The drawing under review shows one solid part. Ordinate dimensions are in mm from its lowest x, y, z. Give positions to 0.01 mm unless a question says otherwise; leave off trailing zeros. Loops run counter-clockwise (first coordinate to the right, second up) from the corner with the lowest first, then second, coordinate; pieces in that order, holes last. Notation, with made-up numbers: (43.5, 77) -> (94.5, 77) arc R16 ccw to (94.5, 106) -> close; hole circle Ø1 at (14.25, 33). An arc over 180 degrees is marked (long way). Answer in a Markdown table with one row per item. Add a question column.
(1) For pin 1 (10 mm diameter, centred on y = 212, z = 5.5, fed in from +X); pin 2 (9.5 mm diameter, centred on x = 6.5, z = 10.5, fed in from -Y); pin 3 (9.5 mm diameter, centred on y = 500.5, z = 11, fed in from -X), all flat-tipped, find the tip position at first contact; note any pin that passes through.
(2) Consider section B-B on z = 13.75. Write out the cut boundary in (x, y), then the cut area to 3 significant figures.
(3) For line 1 (Y direction, x = 423, z = 4); line 2 (X direction, y = 518, z = 7); line 3 (X direction, y = 32, z = 7.5), list the stretches that pass through material, from the lowest coordinate up.
(4) Consider section A-A on x = 373.5. Write out the cut boundary in (y, z), then the cut area to 3 significant figures.
(5) Consider section C-C on y = 207. Write out the cut boundary in (x, z).
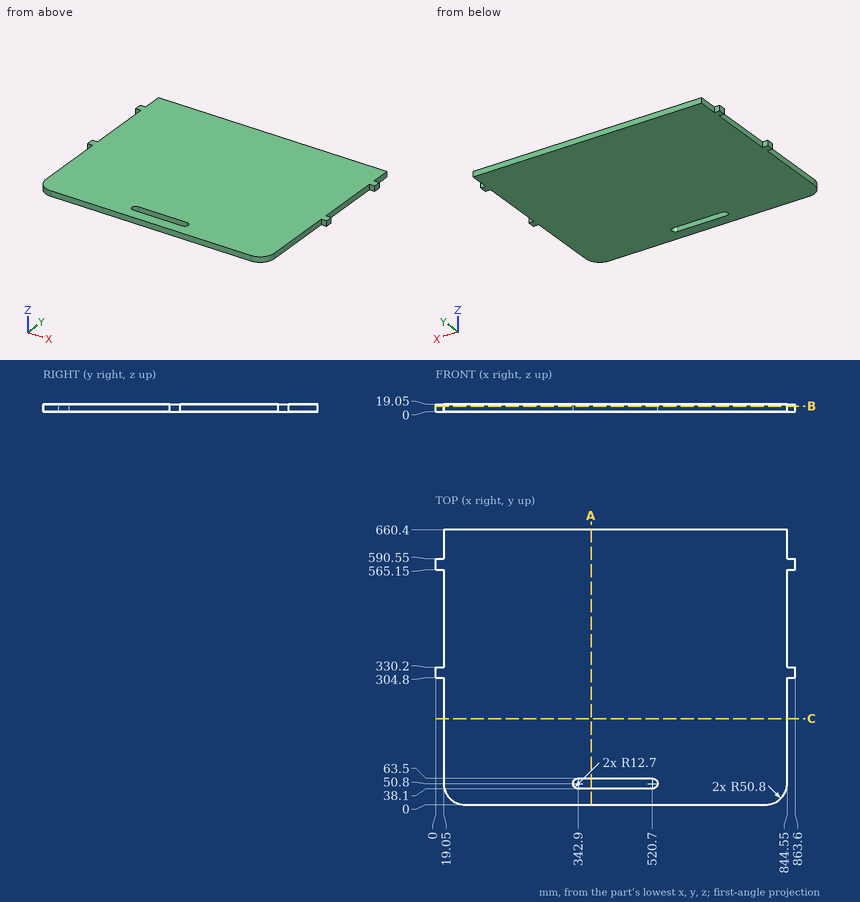
Values follow:
| question | item | result |
|---|---|---|
| 1 | pin 1 | x = 844.55 |
| 1 | pin 2 | y = 304.8 |
| 1 | pin 3 | x = 19.05 |
| 2 | outline | (0, 304.8) -> (19.05, 304.8) -> (19.05, 50.8) arc R50.8 ccw to (69.85, 0) -> (793.75, 0) arc R50.8 ccw to (844.55, 50.8) -> (844.55, 304.8) -> (863.6, 304.8) -> (863.6, 330.2) -> (844.55, 330.2) -> (844.55, 565.15) -> (863.6, 565.15) -> (863.6, 590.55) -> (844.55, 590.55) -> (844.55, 660.4) -> (19.05, 660.4) -> (19.05, 590.55) -> (0, 590.55) -> (0, 565.15) -> (19.05, 565.15) -> (19.05, 330.2) -> (0, 330.2) -> close; hole (342.9, 38.1) -> (520.7, 38.1) arc R12.7 ccw to (520.7, 63.5) -> (342.9, 63.5) arc R12.7 ccw to start |
| 2 | area | 541,000 mm2 |
| 3 | line 1 | 0 to 38.1, 63.5 to 660.4 |
| 3 | line 2 | 19.05 to 844.55 |
| 3 | line 3 | 22.66 to 840.94 |
| 4 | outline | (0, 0) -> (38.1, 0) -> (38.1, 19.05) -> (0, 19.05) -> close; (63.5, 0) -> (660.4, 0) -> (660.4, 19.05) -> (63.5, 19.05) -> close |
| 4 | area | 12,100 mm2 |
| 5 | outline | (19.05, 0) -> (844.55, 0) -> (844.55, 19.05) -> (19.05, 19.05) -> close |
